Geometry: final body of the model. Coordinates: model frame, mm. Coordinates: 2 decimals unless noted, no trailing zeros. Answer in a Markdown table with one row per item.
from build123d import *

# Parameters (mm, degrees)
F1_W      = 133
F1_H      = 111
F1_R      = 10.5
F2_DEPTH  = 2
F2_FACE_W = 133
F2_FACE_H = 111
F2_FACE_R = 10.5
F3_DEPTH  = 0.4
F4_D      = 17


# Not quite as in the source:
# - a feature of the source that left no trace in its solid (it failed there, or was rolled back) is left out


with BuildPart() as f2:
    # F1 (on Top) → F2 (new body)
    with BuildSketch(Plane.XY):
        with Locations((55, 44)):
            Rectangle(F1_W, F1_H)
        Circle(F1_R, mode=Mode.SUBTRACT)
        with Locations((22, 0)):
            Circle(F1_R, mode=Mode.SUBTRACT)
        with Locations((44, 0)):
            Circle(F1_R, mode=Mode.SUBTRACT)
        with Locations((0, 22)):
            Circle(F1_R, mode=Mode.SUBTRACT)
        with Locations((22, 22)):
            Circle(F1_R, mode=Mode.SUBTRACT)
        with Locations((44, 22)):
            Circle(F1_R, mode=Mode.SUBTRACT)
        with Locations((66, 0)):
            Circle(F1_R, mode=Mode.SUBTRACT)
        with Locations((88, 0)):
            Circle(F1_R, mode=Mode.SUBTRACT)
        with Locations((110, 0)):
            Circle(F1_R, mode=Mode.SUBTRACT)
        with Locations((66, 22)):
            Circle(F1_R, mode=Mode.SUBTRACT)
        with Locations((88, 22)):
            Circle(F1_R, mode=Mode.SUBTRACT)
        with Locations((110, 22)):
            Circle(F1_R, mode=Mode.SUBTRACT)
        with Locations((0, 44)):
            Circle(F1_R, mode=Mode.SUBTRACT)
        with Locations((0, 66)):
            Circle(F1_R, mode=Mode.SUBTRACT)
        with Locations((22, 44)):
            Circle(F1_R, mode=Mode.SUBTRACT)
        with Locations((44, 44)):
            Circle(F1_R, mode=Mode.SUBTRACT)
        with Locations((22, 66)):
            Circle(F1_R, mode=Mode.SUBTRACT)
        with Locations((44, 66)):
            Circle(F1_R, mode=Mode.SUBTRACT)
        with Locations((0, 88)):
            Circle(F1_R, mode=Mode.SUBTRACT)
        with Locations((22, 88)):
            Circle(F1_R, mode=Mode.SUBTRACT)
        with Locations((44, 88)):
            Circle(F1_R, mode=Mode.SUBTRACT)
        with Locations((66, 44)):
            Circle(F1_R, mode=Mode.SUBTRACT)
        with Locations((88, 44)):
            Circle(F1_R, mode=Mode.SUBTRACT)
        with Locations((66, 66)):
            Circle(F1_R, mode=Mode.SUBTRACT)
        with Locations((88, 66)):
            Circle(F1_R, mode=Mode.SUBTRACT)
        with Locations((110, 44)):
            Circle(F1_R, mode=Mode.SUBTRACT)
        with Locations((110, 66)):
            Circle(F1_R, mode=Mode.SUBTRACT)
        with Locations((66, 88)):
            Circle(F1_R, mode=Mode.SUBTRACT)
        with Locations((88, 88)):
            Circle(F1_R, mode=Mode.SUBTRACT)
        with Locations((110, 88)):
            Circle(F1_R, mode=Mode.SUBTRACT)
    extrude(amount=F2_DEPTH)

    # F2_face (on face) + F1 (on Top) → F3 (join)
    with BuildSketch(Plane(origin=(55, 44, 2), x_dir=(1, 0, 0), z_dir=(0, 0, 1))):
        Rectangle(F2_FACE_W, F2_FACE_H)
        with Locations((-55, -44)):
            Circle(F2_FACE_R, mode=Mode.SUBTRACT)
        with Locations((-33, -44)):
            Circle(F2_FACE_R, mode=Mode.SUBTRACT)
        with Locations((-11, -44)):
            Circle(F2_FACE_R, mode=Mode.SUBTRACT)
        with Locations((-55, -22)):
            Circle(F2_FACE_R, mode=Mode.SUBTRACT)
        with Locations((-33, -22)):
            Circle(F2_FACE_R, mode=Mode.SUBTRACT)
        with Locations((-11, -22)):
            Circle(F2_FACE_R, mode=Mode.SUBTRACT)
        with Locations((11, -44)):
            Circle(F2_FACE_R, mode=Mode.SUBTRACT)
        with Locations((33, -44)):
            Circle(F2_FACE_R, mode=Mode.SUBTRACT)
        with Locations((55, -44)):
            Circle(F2_FACE_R, mode=Mode.SUBTRACT)
        with Locations((11, -22)):
            Circle(F2_FACE_R, mode=Mode.SUBTRACT)
        with Locations((33, -22)):
            Circle(F2_FACE_R, mode=Mode.SUBTRACT)
        with Locations((55, -22)):
            Circle(F2_FACE_R, mode=Mode.SUBTRACT)
        with Locations((-55, 0)):
            Circle(F2_FACE_R, mode=Mode.SUBTRACT)
        with Locations((-55, 22)):
            Circle(F2_FACE_R, mode=Mode.SUBTRACT)
        with Locations((-33, 0)):
            Circle(F2_FACE_R, mode=Mode.SUBTRACT)
        with Locations((-11, 0)):
            Circle(F2_FACE_R, mode=Mode.SUBTRACT)
        with Locations((-33, 22)):
            Circle(F2_FACE_R, mode=Mode.SUBTRACT)
        with Locations((-11, 22)):
            Circle(F2_FACE_R, mode=Mode.SUBTRACT)
        with Locations((-55, 44)):
            Circle(F2_FACE_R, mode=Mode.SUBTRACT)
        with Locations((-33, 44)):
            Circle(F2_FACE_R, mode=Mode.SUBTRACT)
        with Locations((-11, 44)):
            Circle(F2_FACE_R, mode=Mode.SUBTRACT)
        with Locations((11, 0)):
            Circle(F2_FACE_R, mode=Mode.SUBTRACT)
        with Locations((33, 0)):
            Circle(F2_FACE_R, mode=Mode.SUBTRACT)
        with Locations((11, 22)):
            Circle(F2_FACE_R, mode=Mode.SUBTRACT)
        with Locations((33, 22)):
            Circle(F2_FACE_R, mode=Mode.SUBTRACT)
        with Locations((55, 0)):
            Circle(F2_FACE_R, mode=Mode.SUBTRACT)
        with Locations((55, 22)):
            Circle(F2_FACE_R, mode=Mode.SUBTRACT)
        with Locations((11, 44)):
            Circle(F2_FACE_R, mode=Mode.SUBTRACT)
        with Locations((33, 44)):
            Circle(F2_FACE_R, mode=Mode.SUBTRACT)
        with Locations((55, 44)):
            Circle(F2_FACE_R, mode=Mode.SUBTRACT)
    with BuildSketch(Plane.XY):
        with Locations((0, 88)):
            Circle(F1_R)
        with Locations((22, 88)):
            Circle(F1_R)
        with Locations((44, 88)):
            Circle(F1_R)
        with Locations((66, 88)):
            Circle(F1_R)
        with Locations((88, 88)):
            Circle(F1_R)
        with Locations((110, 88)):
            Circle(F1_R)
        with Locations((110, 66)):
            Circle(F1_R)
        with Locations((88, 66)):
            Circle(F1_R)
        with Locations((66, 66)):
            Circle(F1_R)
        with Locations((44, 66)):
            Circle(F1_R)
        with Locations((22, 66)):
            Circle(F1_R)
        with Locations((0, 66)):
            Circle(F1_R)
        with Locations((22, 44)):
            Circle(F1_R)
        with Locations((0, 44)):
            Circle(F1_R)
        with Locations((44, 44)):
            Circle(F1_R)
        with Locations((66, 44)):
            Circle(F1_R)
        with Locations((88, 44)):
            Circle(F1_R)
        with Locations((110, 44)):
            Circle(F1_R)
        with Locations((110, 22)):
            Circle(F1_R)
        with Locations((88, 22)):
            Circle(F1_R)
        with Locations((66, 22)):
            Circle(F1_R)
        with Locations((44, 22)):
            Circle(F1_R)
        with Locations((22, 22)):
            Circle(F1_R)
        with Locations((0, 22)):
            Circle(F1_R)
        Circle(F1_R)
        with Locations((22, 0)):
            Circle(F1_R)
        with Locations((44, 0)):
            Circle(F1_R)
        with Locations((66, 0)):
            Circle(F1_R)
        with Locations((88, 0)):
            Circle(F1_R)
        with Locations((110, 0)):
            Circle(F1_R)
    extrude(amount=F3_DEPTH)

    # F4 (through all)
    with Locations(Plane(origin=(0, 0, 0), x_dir=(1, 0, 0), z_dir=(0, 0, -1))):
        with Locations((0, -88), (22, -88), (44, -88), (66, -88), (88, -88), (110, -88), (110, -66), (88, -66), (66, -66), (44, -66), (22, -66), (0, -66), (0, -44), (22, -44), (44, -44), (66, -44), (88, -44), (110, -44), (110, -22), (88, -22), (66, -22), (44, -22), (22, -22), (0, -22), (110, 0), (88, 0), (66, 0), (44, 0), (22, 0), (0, 0)):
            Hole(F4_D / 2)


solid = f2.part
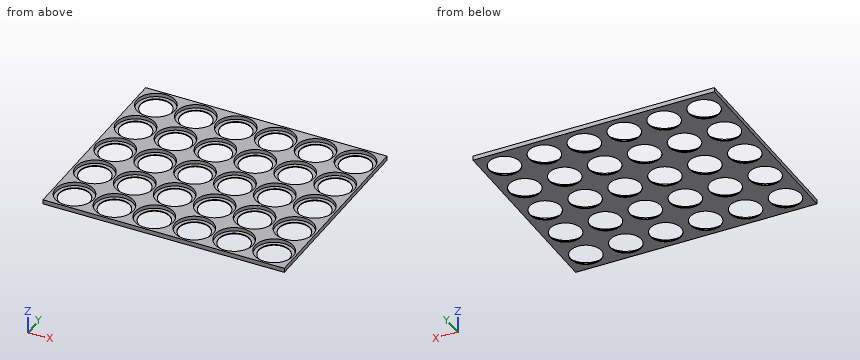
(1) First-contact query: pin 1 Ø10 at (x, y) = (110, 88) entering from +Z; pin 2 Ø19 at (x, y) = (44, 66) entering from +Z. Flat tips, straight axial feed; report the tip coordinate or a pass-through.
Verdict:
| item | result |
|---|---|
| pin 1 | passes through |
| pin 2 | stops at z = 0.4 |
(2) Ray query, probe 1 along Y at (x, z) = (44, 0.2); probe 2 along Y at (x, z) = (22, 1.1); probe 3 along Z at (x, y) = (12.5, 26). Return the intervals inside material, ascending.
Verdict:
| item | result |
|---|---|
| probe 1 | y = -11.5 to -8.5, 8.5 to 13.5, 30.5 to 35.5, 52.5 to 57.5, 74.5 to 79.5, 96.5 to 99.5 |
| probe 2 | y = -11.5 to -10.5, 10.5 to 11.5, 32.5 to 33.5, 54.5 to 55.5, 76.5 to 77.5, 98.5 to 99.5 |
| probe 3 | z = 0 to 0.4 |
(3) Cut plane A-A on z = 1.4. State how many separate pieces and enclosed holes the cut face has, then the cut area to 3 significant figures.
Verdict:
| item | result |
|---|---|
| separate pieces | 1 |
| enclosed holes | 30 |
| area | 4,370 mm² |
